Autodesk Inventor part; units mm, degrees
ref_plane "YZ Plane" through (0, 0, 0) normal (1, 0, 0) x (0, 1, 0)
ref_plane "XZ Plane" through (0, 0, 0) normal (0, 1, 0) x (-1, 0, 0)
ref_plane "XY Plane" through (0, 0, 0) normal (0, 0, 1) x (1, 0, 0)
sketch "Sketch1" plane through (0, 0, 0) normal (0, 1, 0) x (-1, 0, 0)
  circle A0 centre (0, 0) radius 14
  dimension "d0" = 28
extrude "Extrusion1" add sketch "Sketch1" along normal blind 5
sketch "Sketch2" plane through (0, 5, 0) normal (0, 1, 0) x (1, 0, 0)
  circle A0 centre (0, 0) radius 6
  dimension "d3" = 12
extrude "Extrusion2" add sketch "Sketch2" along normal blind 14
sketch "Sketch4" plane through (0, 0, 0) normal (0, -1, 0) x (1, 0, 0)
  circle A0 centre (0, 0) radius 10 construction
  point P0 (0, -10)
  point P1 (0, 10)
  point P2 (-10, 0)
  point P3 (10, 0)
  dimension "d7" = 20
hole "Hole1" at (0, 0, -10) at (0, 0, 10) at (-10, 0, 0) at (10, 0, 0) direction (0, 1, 0) diameter 2.85 end through all counterbore diameter 6 counterbore depth 3.1
sketch "Sketch5" plane through (0, 19, 0) normal (0, 1, 0) x (1, 0, 0)
  point P0 (0, 0)
  point P1 (0, 0)
  dimension "d6" = 20
hole "Hole2" at (0, 19, 0) direction (0, -1, 0) diameter 6 end through all
fillet "Fillet1" radius 0.5 3 edges at (-6, 19, 0) (14, 5, 0) (14, 0, 0)
properties part number "2309HCMUTE-CDT23-BAC_TRUOT" material "Stainless Steel"
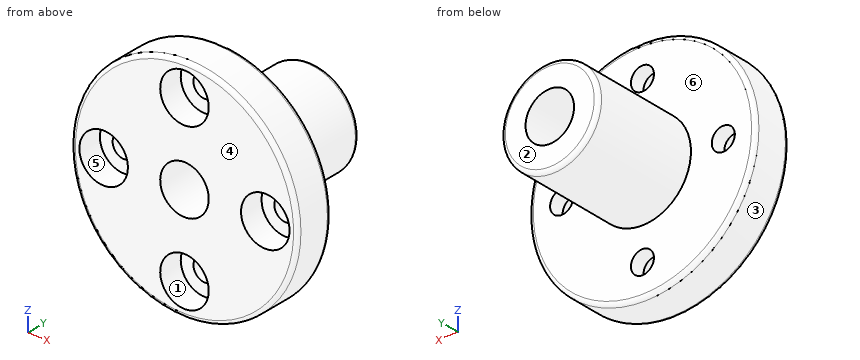
Build history of the part. All positions in model axes, mm. Face numbers are marked on the shaded views. A direction names the side the tool comes from. Give positions to 0.01 mm unless a question says otherwise; leave off trailing zeros. Order: outer loops, then holes, each group sorted by start corner. A loop starts at its lowest first (then second) coordinate and runs counter-clockwise, first axis right, second up. Notation, with made-up numbers: M -36,9.5 L 22,9.5 A13 cw 22,23.5 Z; hole C -20.5,-30.75 d4. An arc over 180 degrees is marked long. Write item = value, one per line. Start each with the question number.
(1) Slice it at B-B on y = 2.25. Write the cut outline in (x, z).
(2) Pin check, flat tips, straight feed: pin 1 Ø5 at (x, z) = (0, 10) entering from +Y; pin 2 Ø2.5 at (x, z) = (10, 0) entering from +Y; pin 3 Ø5.5 at (x, z) = (0, -10) entering from -Y; pin 4 Ø4 at (y, z) = (4.5, -4) entering from -X. Stop position of each tip, or through.
(3) Which spindle directions (+Z, -Z, +X, -X, +Y, -Y) get a long thin tool onto all of the face, cutting with end or side? Do the marked faces 4, 5 and 6. Say none if no direction does.
(4) Slice it at C-C on y = 5.75. Write the cut outline in (x, z).
(5) Probe L1, parallel to Z at x = 0, y = 3.85 (3 decimals); L2, parallel to Z at x = 0, y = 1.25; L3, parallel to Y at x = 0, z = 7.75. List the from-to ranges inside material, lowest first. Write a range as [from, to].
(6) Two-plate mould, pull along Z, no slides. Class the marked faces 1, 2 and 3: released by +Z, released by -Z, zero draft, split by the parting line, or undercut.
(7) Slice it at A-A on z = 0. State how many separate pieces and enclosed holes the cut face has, plus the area to 3 significant figures.
Responses:
q1.outline = C 0,0 d28; hole C -10,0 d6; hole C 0,-10 d6; hole C 0,0 d6; hole C 0,10 d6; hole C 10,0 d6
q2.pin_1 = 5
q2.pin_2 = through
q2.pin_3 = 3.1
q2.pin_4 = -13.86
q3.face_4 = +Z, -Z, +X, -X, -Y
q3.face_5 = -Y
q3.face_6 = +Y
q4.outline = C 0,0 d12; hole C 0,0 d6
q5.L1 = [-14, -11.425], [-8.575, -3], [3, 8.575], [11.425, 14]
q5.L2 = [-14, -13], [-7, -3], [3, 7], [13, 14]
q5.L3 = [3.1, 5]
q6.face_1 = undercut
q6.face_2 = zero draft
q6.face_3 = split by the parting line
q7.separate_pieces = 4
q7.enclosed_holes = 0
q7.area = 146 mm2
